CAD build for the part. Positions are in the model's coordinates, mm. Coordinates: 2 decimals unless noted, no trailing zeros. Loops run counter-clockwise (first coordinate to the right, second up) from the corner with the lowest first, then second, coordinate; pieces in that order, holes last. Notation, with made-up numbers: (0.5, 83.5) - (13.5, 83.5) arc R17 cw to (13.5, 101.5) - close; hole circle Ø1 at (71, 44). An arc over 180 degrees is marked (long way). Put each result on its own line as item: value.
```python
from build123d import *

# Parameters (mm, degrees)
SKETCH1_W           = 100
SKETCH1_H           = 2.5
BOSS_EXTRUDE1_DEPTH = 3
BOSS_EXTRUDE2_DEPTH = 5
FILLET4_R           = 1
FILLET2_R           = 1


with BuildPart() as part:
    # Sketch1 → Boss-Extrude1 (new, symmetric)
    with BuildSketch(Plane(origin=(0, 0, 0), x_dir=(0, 0, -1), z_dir=(1, 0, 0))):
        with Locations((50, -1.25)):
            Rectangle(SKETCH1_W, SKETCH1_H)
    extrude(amount=BOSS_EXTRUDE1_DEPTH, both=True)

    # Sketch2 → Boss-Extrude2 (add, symmetric)
    with BuildSketch(Plane(origin=(0, 0, 0), x_dir=(0, 0, -1), z_dir=(1, 0, 0))):
        with BuildLine():
            Line((0, 0), (-8.840402867, 0))
            Line((-8.840402867, 0), (5.882028998, -8.5))
            ThreePointArc((5.882028998, -8.5), (6.882028998, -8.671572875), (7.882028998, -8.5))
            Line((7.882028998, -8.5), (6.062177826, -3.5))
            Line((6.062177826, -3.5), (0, 0))
        make_face()
    extrude(amount=BOSS_EXTRUDE2_DEPTH, both=True)

    # Fillet4
    # the kernel refuses this fillet: 1 mm, written as the material it adds along each edge
    with BuildSketch(Plane(origin=(-3, -2.5, -4.330127019), x_dir=(0, 0, -1), z_dir=(1, 0, 0))) as fillet4_piece_1:
        with BuildLine():
            CenterArc((2.732050808, -1), FILLET4_R, 90, 90)
            Line((1.732050808, -1), (1.712050808, -1))
            ThreePointArc((1.712050808, -1), (0.856025404, -0.517320508), (-0.01, -0.017320508))
            Line((-0.01, -0.017320508), (0, 0.02))
            Line((0, 0.02), (2.732050808, 0.02))
            Line((2.732050808, 0.02), (2.732050808, 0))
        make_face()
    extrude(amount=6)

    # Fillet2
    fillet2_edges = [part.edges().sort_by_distance(p)[0] for p in [
        (0, 0, 8.840402867),
    ]]
    fillet(fillet2_edges, radius=FILLET2_R)


solid = part.part
```
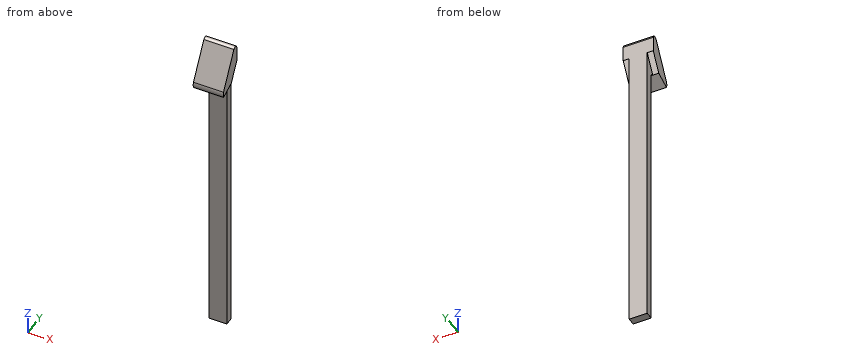
Q1. Slice it at B-B, the plane z = -57. Give the cut face in (x, y).
Determined:
outline: (-3, -2.5) - (3, -2.5) - (3, 0) - (-3, 0) - close
Q2. Slice it at A-A, the plane x = -2. Give the cut face in (y, z), then the cut area to 3 significant figures.
Determined:
outline: (-8.5, -7.88) - (-3.5, -6.06) arc R1 cw to (-2.5, -7.06) - (-2.5, -100) - (0, -100) - (0, 5.11) arc R1 ccw to (-1.87, 5.61) - (-8.5, -5.88) arc R3 ccw to start
area: 302 mm2
Q3. Slice it at C-C, the plane y = -6.75. Give the cut face in (x, z), then the cut area to 3 significant figures.
Determined:
outline: (-5, -7.25) - (5, -7.25) - (5, -2.85) - (-5, -2.85) - close
area: 43.9 mm2
Q4. Pin check, flat tips, straight feed: pin 1 Ø4 at (y, z) = (-2.5, -67.5) entering from -X; pin 2 Ø1.5 at (x, y) = (3, -2) entering from +Z; pin 3 Ø1.8 at (x, z) = (1.5, -48) entering from -Y; pin 4 Ø5 at (x, y) = (-4, -4.5) entering from -Z. Stop position of each tip, or through.
Determined:
pin 1: x = -3
pin 2: z = 6.08
pin 3: y = -2.5
pin 4: z = -100
Q5. Wall check: L1, parallel to X at y = -1.75, z = -4; L2, parallel to Y at x = 2.75, z = -62.5; L3, parallel to Z at x = 0.75, y = -4.25. Give the ranges that are in metal, low to high. Write a range as from..to.
Determined:
L1: -3..3
L2: -2.5..0
L3: -6.34..1.48
